Verification items for this drawing (mm, ordinates from the low corner). A direction names the side the tool comes from. Round coordinates to 2 decimals unless told otherwise and drop trailing zeros. Loops run counter-clockwise (first coordinate to the right, second up) from the corner with the lowest first, then second, coordinate; pieces in that order, holes last. Notation, with made-up numbers: M 34.25,46 L 49.25,46 A23 cw 49.25,64 Z; hole C 13,-40 d6. An arc over 180 degrees is marked long. One line per item, written item: value.
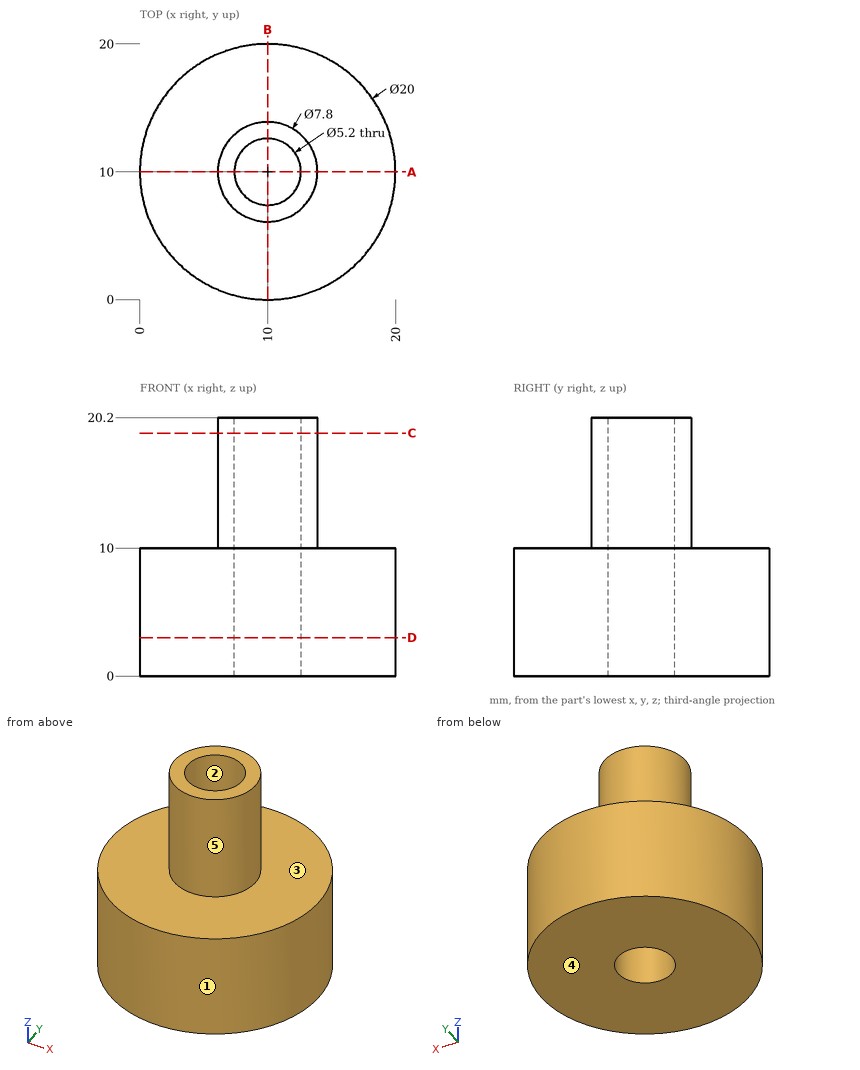
(1) Thickness scan on L1, parallel to Y at x = 10, z = 13.5; L2, parallel to Z at x = 3.5, y = 5.75; L3, parallel to X at y = 11, z = 8.75. Record the ranges inside material, lowest first. Write a range as from..to.
Completed:
L1: y = 6.1..7.4, 12.6..13.9
L2: z = 0..10
L3: x = 0.05..7.6, 12.4..19.95
(2) Sectioned sample at A-A on y = 10. Enter the section's corners in (x, z).
Completed:
outline: M 0,0 L 7.4,0 L 7.4,20.2 L 6.1,20.2 L 6.1,10 L 0,10 Z; M 12.6,0 L 20,0 L 20,10 L 13.9,10 L 13.9,20.2 L 12.6,20.2 Z
(3) Sectioned sample at D-D on z = 3. Enter the section's corners in (x, y).
Completed:
outline: C 10,10 d20; hole C 10,10 d5.2
(4) Sectioned sample at C-C on z = 19. Enter the section's corners in (x, y), and give its area (3 significant figures).
Completed:
outline: C 10,10 d7.8; hole C 10,10 d5.2
area: 26.5 mm^2
(5) Depth check by flat-ended pin: pin 1 Ø4 at (y, z) = (5, 13.5) entering from -X; pin 2 Ø5 at (y, z) = (17.5, 2.5) entering from -X; pin 3 Ø1 at (y, z) = (9, 9.5) entering from +X; pin 4 Ø3 at (x, y) = (10, 10) entering from -Z. Enter the tip coordinate at first touch or a pass-through.
Completed:
pin 1: stops at x = 7.51
pin 2: stops at x = 1.34
pin 3: stops at x = 19.99
pin 4: passes through
(6) Mould release check, pull along Y, two halves, no side actions. Record for the marked faces 1, 2 and 3: +Y half, -Y half, draft (parallel to the pull), parting line (faces both ways), or undercut.
Completed:
face 1: parting line
face 2: undercut
face 3: draft
(7) Tool access check on the marked faces 4 and 5. Record the directions out of +Z, -Z, +X, -X, +Y, -Y that give a thin tool (end or side, any length) a straight path to the whole face; none if there is none.
Completed:
face 4: -Z, +X, -X, +Y, -Y
face 5: +Z
